Part print with two shaded views. Sizes in mm from the minimum x, y, z corner. Give positions to 0.01 mm unless a question says otherwise; leave off trailing zeros. Write each loop counter-clockwise with the first axis right and the second up, starting at its lowest first coordinate (ties: lowest second). Pieces come first, ordered by that corner, then holes. Notation, with made-up numbers: M 70,80.25 L 90,80.25 A24 cw 90,94.25 Z; hole C 27,-32 d10. An arc over 180 degrees is marked long. Return JSON: item names as keys, results as strings. Group by question number.
Q1. Band-saw the part on A-A, the plane y = 0.85. Give the cut face in (x, z).
Q2. Band-saw the part on B-B, the plane x = 3.5. Give the cut face in (y, z), then the cut area to 3 significant figures.
Q3. Band-saw the part on C-C, the plane z = 14.74. Give the cut face in (x, y).
Q4. Wall check: probe 1 along X at (y, z) = (0.7, 4.58); probe 2 along X at (y, z) = (1, 14.5). Give the ranges that are in metal, low to high.
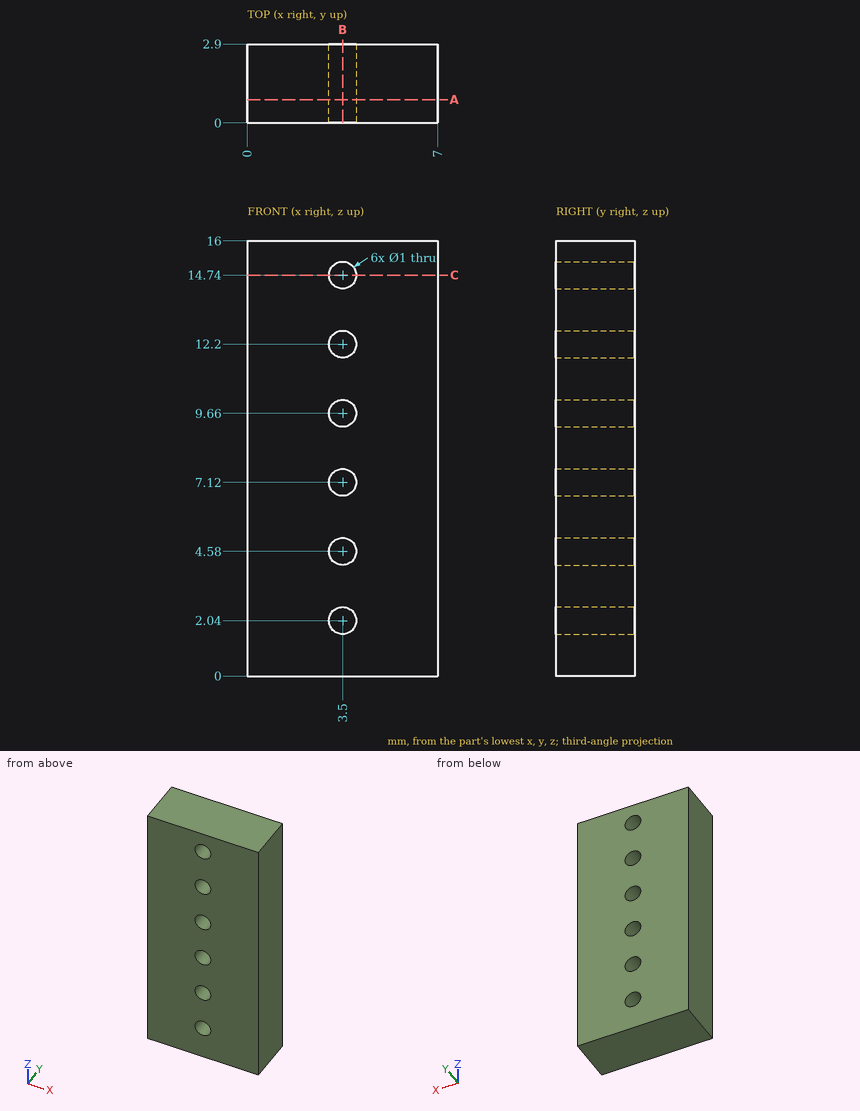
From the geometry:
{
 "1": {"outline": "M 0,0 L 7,0 L 7,16 L 0,16 Z; hole C 3.5,2.04 d1; hole C 3.5,4.58 d1; hole C 3.5,7.12 d1; hole C 3.5,9.66 d1; hole C 3.5,12.2 d1; hole C 3.5,14.74 d1"},
 "2": {"outline": "M 0,0 L 2.9,0 L 2.9,1.54 L 0,1.54 Z; M 0,2.54 L 2.9,2.54 L 2.9,4.08 L 0,4.08 Z; M 0,5.08 L 2.9,5.08 L 2.9,6.62 L 0,6.62 Z; M 0,7.62 L 2.9,7.62 L 2.9,9.16 L 0,9.16 Z; M 0,10.16 L 2.9,10.16 L 2.9,11.7 L 0,11.7 Z; M 0,12.7 L 2.9,12.7 L 2.9,14.24 L 0,14.24 Z; M 0,15.24 L 2.9,15.24 L 2.9,16 L 0,16 Z", "area": "29.0 mm^2"},
 "3": {"outline": "M 0,0 L 3,0 L 3,2.9 L 0,2.9 Z; M 4,0 L 7,0 L 7,2.9 L 4,2.9 Z"},
 "4": {"probe 1": "x = 0 to 3, 4 to 7", "probe 2": "x = 0 to 3.06, 3.94 to 7"}
}
